from build123d import *

# Parameters (mm, degrees)
SKETCH1_W           = 300
SKETCH1_H           = 200
BOSS_EXTRUDE1_DEPTH = 127
FILLET1_R           = 10
SHELL1_T            = -2


with BuildPart() as part:
    # Sketch1 → Boss-Extrude1 (new body)
    with BuildSketch(Plane(origin=(0, 0, 0), x_dir=(1, 0, 0), z_dir=(0, 1, 0))):
        Rectangle(SKETCH1_W, SKETCH1_H)
    extrude(amount=BOSS_EXTRUDE1_DEPTH)

    # Fillet1
    fillet1_edges = [part.edges().sort_by_distance(p)[0] for p in [
        (150, 0, 0),
        (0, 0, 100),
        (-150, 0, 0),
        (0, 0, -100),
        (150, 63.5, -100),
        (150, 63.5, 100),
        (-150, 63.5, 100),
        (-150, 63.5, -100),
    ]]
    fillet(fillet1_edges, radius=FILLET1_R)

    # Shell1
    shell1_openings = [part.faces().sort_by_distance(p)[0] for p in [
        (0, 127, 0),
    ]]
    offset(amount=SHELL1_T, openings=shell1_openings, kind=Kind.INTERSECTION)


solid = part.part
Here's how the part is built. I have some questions about the finished solid (model axes, mm). A direction names the side the tool comes from. Round coordinates to 2 decimals unless told otherwise and drop trailing zeros. Order: outer loops, then holes, each group sorted by start corner. A loop starts at its lowest first (then second) coordinate and runs counter-clockwise, first axis right, second up. Notation, with made-up numbers: M -22.5,-20 L -2.5,-20 A12 cw -2.5,-14 Z; hole C -22.75,15.25 d2. An arc over 180 degrees is marked long. Return JSON: item names as keys, results as strings. Group by question number.
1. Please list where these lines run through material, in increasing order: probe 1 along X at (y, z) = (91, -51); probe 2 along Z at (x, y) = (119, 90); probe 3 along Z at (x, y) = (-138, 9).
2. If we section it at C-C on y = 48.5: List the corners of the cut face in (x, z) for me, then the cut area to 3 significant figures.
3. On a 3-axis mill with a long thin cutter (end or side, diameter ignored), from which of +Z, -Z, +X, -X, +Y, -Y can I reach the whole of each face in a straight line? I mean faces 5 (the face through (148, 68, 1)), 6 (the face through (147.15, 3.01, -1.26)). Say none if no direction works.
4. If we mould it in two halves opening along X, with no side actions, what happens to faces 1 (the face through (146.99, 69.32, 97.15)), 2 (the face through (1.96, 4.406, -95.719)), 3 (the face through (1.96, 3.01, 97.15)), 4 (the face through (1.96, 4.406, 95.719))? For each: pulls with the +X half, pulls with the -X half, needs draft (parallel to the pull), parting line crosses it, or undercut.
5. I'm going to push a flat-ended pin straight in: pin 1 Ø1.5 at (x, z) = (5, 3) entering from +Y. Where does the tip first touch, or does it pass through?
6. If we section it at B-B on z = 66: List the corners of the cut face in (x, y) for me, then the cut area to 3 significant figures.
7. If we section it at A-A on x = 126: List the corners of the cut face in (y, z) for me, then the cut area to 3 significant figures.
Reply:
{
 "1": {"probe 1": "-150 to -148, 148 to 150", "probe 2": "-100 to -98, 98 to 100", "probe 3": "-99.95 to -97.94, 97.94 to 99.95"},
 "2": {"outline": "M -150,-90 A10 ccw -140,-100 L 140,-100 A10 ccw 150,-90 L 150,90 A10 ccw 140,100 L -140,100 A10 ccw -150,90 Z; hole M -148,-90 A8 ccw -140,-98 L 140,-98 A8 ccw 148,-90 L 148,90 A8 ccw 140,98 L -140,98 A8 ccw -148,90 Z", "area": "1,950 mm^2"},
 "3": {"face 5": "+Y", "face 6": "+Z, -Z, +X, -Y"},
 "4": {"face 1": "pulls with the +X half", "face 2": "undercut", "face 3": "needs draft", "face 4": "undercut"},
 "5": {"pin 1": "y = 2"},
 "6": {"outline": "M -150,10 A10 ccw -140,0 L 140,0 A10 ccw 150,10 L 150,127 L 148,127 L 148,10 A8 cw 140,2 L -140,2 A8 cw -148,10 L -148,127 L -150,127 Z", "area": "1,080 mm^2"},
 "7": {"outline": "M 0,-90 A10 ccw 10,-100 L 127,-100 L 127,-98 L 10,-98 A8 cw 2,-90 L 2,90 A8 cw 10,98 L 127,98 L 127,100 L 10,100 A10 ccw 0,90 Z", "area": "885 mm^2"}
}
